from build123d import *

# Parameters (mm, degrees)
F0_W        = 34.544
F0_H        = 19
F1_DEPTH    = 3.81
F3_R        = 2.667
F4_DEPTH    = 10.16
F6_DEPTH    = 19.001
F7_W        = 34.544
F7_H        = 1.778
F8_DEPTH    = 4.826
F9_T1_DEPTH = 30.226
F9_T3_DEPTH = 29.21


# Not quite as in the source:
# - a fillet or chamfer that OpenCascade refuses, or shapes differently, is made with other operations: its cross-section is extruded or revolved along the edge and cut away or added


with BuildPart() as f1:
    # F0 (on Top) → F1 (new body)
    with BuildSketch(Plane.XY):
        Rectangle(F0_W, F0_H)
    extrude(amount=F1_DEPTH)

    # F3 (on face) → F4 (cut)
    with BuildSketch(Plane.XY.offset(3.81)):
        with Locations((-12.827, -5.055)):
            Circle(F3_R)
        with Locations((12.827, -5.055)):
            Circle(F3_R)
    extrude(amount=-F4_DEPTH, mode=Mode.SUBTRACT)

    # F5 (on face) → F6 (cut, through all)
    with BuildSketch(Plane.XZ.offset(9.5)):
        Polygon((-17.78, 3.302), (-17.272, 3.81), (-18.288, 3.81), align=None)
        Polygon((-16.764, 3.302), (-16.256, 3.81), (-17.272, 3.81), align=None)
        Polygon((-15.748, 3.302), (-15.24, 3.81), (-16.256, 3.81), align=None)
        Polygon((-14.732, 3.302), (-14.224, 3.81), (-15.24, 3.81), align=None)
        Polygon((-13.716, 3.302), (-13.208, 3.81), (-14.224, 3.81), align=None)
        Polygon((-12.7, 3.302), (-12.192, 3.81), (-13.208, 3.81), align=None)
        Polygon((-11.684, 3.302), (-11.176, 3.81), (-12.192, 3.81), align=None)
        Polygon((-10.668, 3.302), (-10.16, 3.81), (-11.176, 3.81), align=None)
        Polygon((-9.652, 3.302), (-9.144, 3.81), (-10.16, 3.81), align=None)
        Polygon((-8.636, 3.302), (-8.128, 3.81), (-9.144, 3.81), align=None)
        Polygon((-7.62, 3.302), (-7.112, 3.81), (-8.128, 3.81), align=None)
        Polygon((-6.604, 3.302), (-6.096, 3.81), (-7.112, 3.81), align=None)
        Polygon((-5.588, 3.302), (-5.08, 3.81), (-6.096, 3.81), align=None)
        Polygon((-4.572, 3.302), (-4.064, 3.81), (-5.08, 3.81), align=None)
        Polygon((-3.556, 3.302), (-3.048, 3.81), (-4.064, 3.81), align=None)
        Polygon((-2.54, 3.302), (-2.032, 3.81), (-3.048, 3.81), align=None)
        Polygon((-1.524, 3.302), (-1.016, 3.81), (-2.032, 3.81), align=None)
        Polygon((-0.508, 3.302), (0, 3.81), (-1.016, 3.81), align=None)
        Polygon((0.508, 3.302), (1.016, 3.81), (0, 3.81), align=None)
        Polygon((1.524, 3.302), (2.032, 3.81), (1.016, 3.81), align=None)
        Polygon((2.54, 3.302), (3.048, 3.81), (2.032, 3.81), align=None)
        Polygon((3.556, 3.302), (4.064, 3.81), (3.048, 3.81), align=None)
        Polygon((4.572, 3.302), (5.08, 3.81), (4.064, 3.81), align=None)
        Polygon((5.588, 3.302), (6.096, 3.81), (5.08, 3.81), align=None)
        Polygon((6.604, 3.302), (7.112, 3.81), (6.096, 3.81), align=None)
        Polygon((7.62, 3.302), (8.128, 3.81), (7.112, 3.81), align=None)
        Polygon((8.636, 3.302), (9.144, 3.81), (8.128, 3.81), align=None)
        Polygon((9.652, 3.302), (10.16, 3.81), (9.144, 3.81), align=None)
        Polygon((10.668, 3.302), (11.176, 3.81), (10.16, 3.81), align=None)
        Polygon((11.684, 3.302), (12.192, 3.81), (11.176, 3.81), align=None)
        Polygon((12.7, 3.302), (13.208, 3.81), (12.192, 3.81), align=None)
        Polygon((13.716, 3.302), (14.224, 3.81), (13.208, 3.81), align=None)
        Polygon((14.732, 3.302), (15.24, 3.81), (14.224, 3.81), align=None)
        Polygon((15.748, 3.302), (16.256, 3.81), (15.24, 3.81), align=None)
        Polygon((16.764, 3.302), (17.272, 3.81), (16.256, 3.81), align=None)
    extrude(amount=-F6_DEPTH, mode=Mode.SUBTRACT)

    # F7 (on face) → F8 (join)
    with BuildSketch(Plane(origin=(0, 0, 0), x_dir=(1, 0, 0), z_dir=(0, 0, -1))):
        with Locations((0, 8.611)):
            Rectangle(F7_W, F7_H)
    extrude(amount=-F8_DEPTH)

    # F9: fillet of radius 5.08 on 4 edges, made by hand

    # F9_s2 → F9_t1 (cut)
    with BuildSketch(Plane.XY.offset(-12.7)):
        with BuildLine():
            ThreePointArc((12.192, -9.5), (15.7841024484, -8.0121024484), (17.272, -4.42))
            Line((17.272, -4.42), (17.272, -9.5))
            Line((17.272, -9.5), (12.192, -9.5))
        make_face()
        with BuildLine():
            ThreePointArc((-12.192, -9.5), (-15.7841024484, -8.0121024484), (-17.272, -4.42))
            Line((-17.272, -4.42), (-17.272, -9.5))
            Line((-17.272, -9.5), (-12.192, -9.5))
        make_face()
    extrude(amount=F9_T1_DEPTH, mode=Mode.SUBTRACT)

    # F9_s4 → F9_t3 (cut)
    with BuildSketch(Plane.XY.offset(-12.7)):
        with BuildLine():
            ThreePointArc((17.272, 4.42), (15.7841024484, 8.0121024484), (12.192, 9.5))
            Line((12.192, 9.5), (17.272, 9.5))
            Line((17.272, 9.5), (17.272, 4.42))
        make_face()
        with BuildLine():
            ThreePointArc((-12.192, 9.5), (-15.7841024484, 8.0121024484), (-17.272, 4.42))
            Line((-17.272, 4.42), (-17.272, 9.5))
            Line((-17.272, 9.5), (-12.192, 9.5))
        make_face()
    extrude(amount=F9_T3_DEPTH, mode=Mode.SUBTRACT)


solid = f1.part
Geometry: final body of the model. Coordinates: model frame, mm. Coordinates: 2 decimals unless noted, no trailing zeros. Order: outer loops, then holes, each group sorted by start corner. A loop starts at its lowest first (then second) coordinate and runs counter-clockwise, first axis right, second up. Notation, with made-up numbers: M 61,42.5 L 87,42.5 A29 cw 87,68.5 Z; hole C 63,85 d8. An arc over 180 degrees is marked long. One line per question, with ' | ' between items. Start each with the question number.
Item 1: Ray query, probe 1 along X at (y, z) = (-5.5, 0.7); probe 2 along Y at (x, z) = (12, 3.7); probe 3 along Y at (x, z) = (-13.5, 2.75). Return the intervals inside material, ascending. Write a range as [from, to].
Item 2: Cut plane A-A, the plane z = 4.3. Return the cut outline in (x, y), then the cut area to 3 significant figures.
Item 3: Draft query along Y for faces 1 (the cylindrical face through (15.29, -6.08, 1.93)), 2 (the flat face through (0, -7.722, 4)), 3 (the cylindrical face through (-11.4, -2.8, 1.9)), 4 (the flat face through (-17.272, 0, 2)). Return one class per face: released by +Y, released by -Y, zero draft, split by the parting line, or undercut.
Item 4: Pin query (flat end, axial travel): pin 1 Ø1.5 at (x, y) = (12, -2.5) entering from +Z; pin 2 Ø2 at (y, z) = (-7, 3) entering from -X; pin 3 Ø0.5 at (x, z) = (5.5, 4) entering from +Y. Return the tip coordinate at first contact, or that it passes through.
A:
1) probe 1: x = [-17.16, -15.46], [-10.2, 10.2], [15.46, 17.16] | probe 2: y = [-9.5, -7.72] | probe 3: y = [-9.33, -7.64], [-2.47, 9.33]
2) outline: M -16.05,-7.72 A5.08 ccw -12.19,-9.5 L 12.19,-9.5 A5.08 ccw 16.05,-7.72 Z | area: 52.9 mm2
3) face 1: undercut | face 2: released by +Y | face 3: undercut | face 4: zero draft
4) pin 1: stops at z = 3.81 | pin 2: stops at x = -17.02 | pin 3: stops at y = -7.72
